```python
from build123d import *

# Parameters (mm, degrees)
ESTRUSIONE_ESTRUSIONE1_DEPTH = 10
SCHIZZO2_R                   = 1.75
TAGLIO_ESTRUSIONE1_DEPTH     = 21.645708387


with BuildPart() as part:
    # Schizzo1 → Estrusione-Estrusione1 (new, symmetric)
    with BuildSketch(Plane.XY):
        Polygon((11, 9), (11, 10), (-11, 10), (-11, 9), (-15.041451884, 2), (-15.041451884, 0), (15.041451884, 0), (15.041451884, 2), align=None)
    extrude(amount=ESTRUSIONE_ESTRUSIONE1_DEPTH, both=True)

    # Schizzo2 → Taglio-Estrusione1 (cut, through all)
    with BuildSketch(Plane(origin=(0, 10, 0), x_dir=(1, 0, 0), z_dir=(0, 1, 0))):
        with Locations(Location((7.25, 6.25, 0), (0, 0, 180))):
            Circle(SCHIZZO2_R)
        with Locations(Location((-7.25, 6.25, 0), (0, 0, 180))):
            Circle(SCHIZZO2_R)
        with Locations(Location((-7.25, -6.25, 0), (0, 0, 180))):
            Circle(SCHIZZO2_R)
        with Locations(Location((7.25, -6.25, 0), (0, 0, 180))):
            Circle(SCHIZZO2_R)
    extrude(amount=-TAGLIO_ESTRUSIONE1_DEPTH, mode=Mode.SUBTRACT)


solid = part.part
```
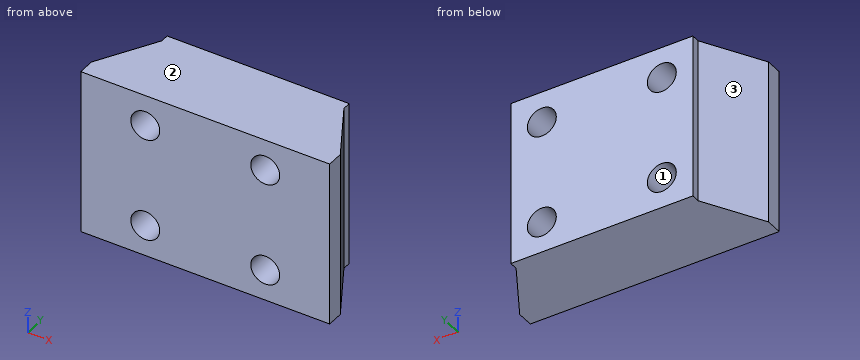
Geometry check sheet. Reference: the model listing, model coordinates, mm. Face numbers are marked on the shaded views. Coordinates: 2 decimals unless noted, no trailing zeros. Loops run counter-clockwise (first coordinate to the right, second up) from the corner with the lowest first, then second, coordinate; pieces in that order, holes last.
Item 1: Sectioned sample at B-B, the plane z = -6.25. Record the boundary of the cut face in (x, y).
Item 2: Release check for a two-part mould opening along X. For the marked faces 1, 2 and 3 record: released by +X, released by -X, zero draft, split by the parting line, or undercut.
Item 3: Sectioned sample at A-A, the plane y = 0.5. Record the boundary of the cut face in (x, z).
Item 4: Thickness scan on line 1 (Z direction, x = -7.25, y = 8); line 2 (Z direction, x = 8.5, y = 4.25); line 3 (X direction, y = 4.5, z = 5). Record the ranges inside material, lowest first.
Item 5: Sectioned sample at D-D, the plane z = -8.5. Record the boundary of the cut face in (x, y).
Item 6: Sectioned sample at C-C, the plane x = -7.25. Record the boundary of the cut face in (y, z).
Item 7: Go/stop test with flat-tipped pins: pin 1 Ø0.5 at (y, z) = (9.5, 0.5) entering from +X; pin 2 Ø0.8 at (y, z) = (9.5, -3.5) entering from -X. Record where each tip stops, or that it passes through.
Check result:
1. outline: (-15.04, 0) - (-9, 0) - (-9, 10) - (-11, 10) - (-11, 9) - (-15.04, 2) - close; (-5.5, 0) - (5.5, 0) - (5.5, 10) - (-5.5, 10) - close; (9, 0) - (15.04, 0) - (15.04, 2) - (11, 9) - (11, 10) - (9, 10) - close
2. face 1: undercut
2. face 2: zero draft
2. face 3: released by -X
3. outline: (-15.04, -10) - (15.04, -10) - (15.04, 10) - (-15.04, 10) - close; hole circle Ø3.5 at (-7.25, -6.25); hole circle Ø3.5 at (-7.25, 6.25); hole circle Ø3.5 at (7.25, -6.25); hole circle Ø3.5 at (7.25, 6.25)
4. line 1: z = -10 to -8, -4.5 to 4.5, 8 to 10
4. line 2: z = -10 to -7.47, -5.03 to 5.03, 7.47 to 10
4. line 3: x = -13.6 to -8.47, -6.03 to 6.03, 8.47 to 13.6
5. outline: (-15.04, 0) - (15.04, 0) - (15.04, 2) - (11, 9) - (11, 10) - (-11, 10) - (-11, 9) - (-15.04, 2) - close
6. outline: (0, -10) - (10, -10) - (10, -8) - (0, -8) - close; (0, -4.5) - (10, -4.5) - (10, 4.5) - (0, 4.5) - close; (0, 8) - (10, 8) - (10, 10) - (0, 10) - close
7. pin 1: stops at x = 11
7. pin 2: stops at x = -11
